For this review, take the finished solid that the model builds, in its own axes (mm). Face numbers are marked on the shaded views. A direction names the side the tool comes from. Coordinates: 2 decimals unless noted, no trailing zeros. Write each loop counter-clockwise with the first axis right and the second up, starting at its lowest first coordinate (ties: lowest second). Pieces come first, ordered by that corner, then holes.
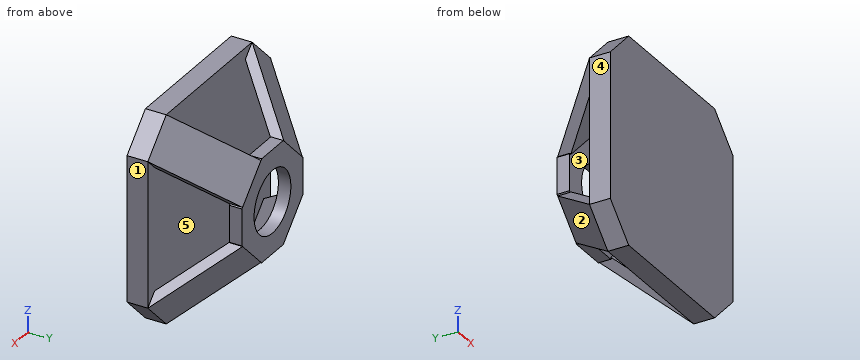
```python
from build123d import *
from build123d.topology import SkipClean

# Parameters (mm, degrees)
SKETCH1_W               = 20
SKETCH1_H               = 20
BOSS_EXTRUDE1_DEPTH     = 2
CHAMFER1_SIZE           = 3
EXTRUDE_THIN1_DEPTH     = 14.142136
CUT_EXTRUDE1_DEPTH      = 9.899495
CIRPATTERN5_START       = -2.121320344
CIRPATTERN5_DEPTH       = 4.242640688
CIRPATTERN5_START_2     = 12.02081528
CIRPATTERN5_2_DEPTH     = 4.242640687
CIRPATTERN5_START_3     = 2.121320344
CIRPATTERN5_3_OUTLINE_W = 4.242640688
CIRPATTERN5_3_OUTLINE_H = 2
CIRPATTERN5_3_DEPTH     = 9.899494936
SKETCH7_W               = 24.04163056
SKETCH7_H               = 24.04163056
CUT_EXTRUDE2_DEPTH      = 4
BOSS_EXTRUDE2_DEPTH     = 1.2
CHAMFER5_SIZE           = 2.5
CUT_EXTRUDE3_REACH      = 31.418
SKETCH10_R              = 3


with BuildPart() as part:
    # Sketch1 → Boss-Extrude1 (new body)
    with BuildSketch(Plane(origin=(0, 0, 0), x_dir=(1, 0, 0), z_dir=(0, 1, 0))):
        with Locations((10, 10)):
            Rectangle(SKETCH1_W, SKETCH1_H)
    extrude(amount=BOSS_EXTRUDE1_DEPTH)

    # Chamfer1
    chamfer1_edges = [part.edges().sort_by_distance(p)[0] for p in [
        (0, 1, -20),
        (20, 1, -20),
        (20, 1, 0),
        (0, 1, 0),
    ]]
    chamfer(chamfer1_edges, length=CHAMFER1_SIZE)



with BuildPart() as body_2:
    # Sketch3 → Extrude-Thin1 (new body)
    with BuildSketch(Plane(origin=(-8.5, 0, -8.5), x_dir=(-0.7071067811865488, 0, 0.7071067811865464), z_dir=(-0.7071067811865464, 0, -0.7071067811865488))):
        Polygon((-2.121320344, 2), (-14.142135624, 12.086661668), (-14.784923233, 11.320617225), (-2.764107953, 1.233955557), align=None)
    extrude(amount=-EXTRUDE_THIN1_DEPTH)

    # Sketch5 → Cut-Extrude1 (cut)
    with BuildSketch(Plane(origin=(-8.5, 0, -8.5), x_dir=(-0.7071067811865488, 0, 0.7071067811865462), z_dir=(-0.7071067811865462, 0, -0.7071067811865488))):
        Polygon((-2.121320344, 2), (-14.142135624, 12.086661668), (-14.784923233, 11.320617225), (-2.764107953, 1.233955557), align=None)
    extrude(amount=-CUT_EXTRUDE1_DEPTH, mode=Mode.SUBTRACT)


with BuildPart() as part_1:
    # CirPattern5: read off the stored shape, not the designer's step
    with SkipClean():  # the faces are left unmerged after this step: merging them gives an invalid solid
        add(part.part)

        add(body_2.part)  # CirPattern5 merges body 2
        # CirPattern5 outline → CirPattern5 (add)
        with BuildSketch(Plane(origin=(0, 0, 0), x_dir=(0.707106781186549, 0, -0.707106781186546), z_dir=(0.707106781186546, 0, 0.707106781186549)).offset(CIRPATTERN5_START)):
            Polygon((14.142135624, 10.781254379), (24.607227077, 2), (26.162950904, 2), (16.263455967, 10.306662551), (14.142135624, 12.086661668), (14.784923233, 11.320617225), align=None)
        extrude(amount=CIRPATTERN5_DEPTH)

    # CirPattern5 2 outline → CirPattern5 2 (add)
    with SkipClean():  # the faces are left unmerged after this step: merging them gives an invalid solid
        with BuildSketch(Plane(origin=(0, 0, 0), x_dir=(0.7071067811865541, 0, 0.707106781186541), z_dir=(0.707106781186541, 0, -0.707106781186554)).offset(CIRPATTERN5_START_2)):
            Polygon((0, -10.781254379), (-10.465091453, -2), (-12.02081528, -2), (-2.121320344, -10.30666255), (0, -12.086661668), (2.121320344, -10.30666255), (12.02081528, -2), (10.465091453, -2), align=None)
        extrude(amount=CIRPATTERN5_2_DEPTH)

    # CirPattern5 3 outline → CirPattern5 3 (add)
    with SkipClean():  # the faces are left unmerged after this step: merging them gives an invalid solid
        with BuildSketch(Plane(origin=(0, 0, 0), x_dir=(0.7071067811865541, 0, 0.707106781186541), z_dir=(0.707106781186541, 0, -0.707106781186554)).offset(CIRPATTERN5_START_3)):
            with Locations((0, -1)):
                Rectangle(CIRPATTERN5_3_OUTLINE_W, CIRPATTERN5_3_OUTLINE_H)
        extrude(amount=CIRPATTERN5_3_DEPTH)

    # Sketch7 → Cut-Extrude2 (cut)
    with BuildSketch(Plane(origin=(0, 12.086661668, 0), x_dir=(-0.7071067811865464, 0, -0.7071067811865488), z_dir=(0, 1, 0))):
        with Locations((0, -14.142135624)):
            Rectangle(SKETCH7_W, SKETCH7_H)
    extrude(amount=-CUT_EXTRUDE2_DEPTH, mode=Mode.SUBTRACT)

    # Sketch9 → Boss-Extrude2 (add)
    with BuildSketch(Plane(origin=(0, 8.086661668, 0), x_dir=(1, 0, 0), z_dir=(0, 1, 0))):
        Polygon((10, 16.741576375), (3.258423625, 10), (10, 3.258423625), (16.741576375, 10), align=None)
    extrude(amount=-BOSS_EXTRUDE2_DEPTH)

    # Chamfer5
    chamfer5_edges = [part_1.edges().sort_by_distance(p)[0] for p in [
        (10, 7.486661668, -3.258423625),
        (10, 7.486661668, -16.741576375),
        (16.741576375, 7.486661668, -10),
        (3.258423625, 7.486661668, -10),
    ]]
    chamfer(chamfer5_edges, length=CHAMFER5_SIZE)

    # Sketch10 → Cut-Extrude3 (cut, up to next)
    with BuildSketch(Plane(origin=(0, 8.086661668, 0), x_dir=(1, 0, 0), z_dir=(0, 1, 0)), mode=Mode.PRIVATE) as cut_extrude3_sk1:
        with Locations(Location((10, 10, 0), (0, 0, 270))):
            Circle(SKETCH10_R)
    cut_extrude3_tool1 = extrude(cut_extrude3_sk1.sketch, amount=-CUT_EXTRUDE3_REACH, mode=Mode.PRIVATE) & part_1.part
    add(cut_extrude3_tool1.solids().sort_by_distance((10, 8.086662, -10))[0], mode=Mode.SUBTRACT)


solid = part_1.part
```
Q1. Add section B-B (x = 10). State the section outline as (y, z) points, then the cut area to 3 significant figures.
Ans:
outline: (0, -20) - (2, -20) - (2, 0) - (0, 0) - close; (6.89, -14.97) - (8.09, -14.97) - (8.09, -13) - (6.89, -13) - close; (6.89, -7) - (8.09, -7) - (8.09, -5.03) - (6.89, -5.03) - close
area: 44.7 mm2
Q2. Draft analysis for pull direction Y (two halves, no side actions). For the marked faces 1, 2 and 3, state which applies: +Y half, -Y half, draft (parallel to the pull), parting line (faces both ways), or undercut.
Ans:
face 1: draft
face 2: +Y half
face 3: undercut
Q3. Add section D-D (z = -3.75). State the section outline as (x, y) points, then the cut area to 3 significant figures.
Ans:
outline: (0, 0) - (20, 0) - (20, 2) - (19.25, 2) - (19.25, 2.89) - (13.25, 6.45) - (13.25, 5.14) - (18.55, 2) - (1.45, 2) - (6.75, 5.14) - (6.75, 6.45) - (0.75, 2.89) - (0.75, 2) - (0, 2) - close
area: 55.4 mm2
Q4. Tool access review of the marked faces 4 and 5: name each direction out of +Z, -Z, +X, -X, +Y, -Y from which nothing blocks a thin tool from reaching the whole face with its end or side.
Ans:
face 4: +Z, -Z, -X, +Y, -Y
face 5: none
Q5. For probe 1 along X at (y, z) = (7.65, -10); probe 2 along Y at (x, z) = (10, -14); probe 3 along Y at (x, z) = (2, -8.75), list the stretches that pass through material, from the lowest coordinate up.
Ans:
probe 1: x = 5.03 to 7, 13 to 14.97
probe 2: y = 0 to 2, 6.89 to 8.09
probe 3: y = 0 to 2
Q6. Add section A-A (z = -10). State the section outline as (x, y) points.
Ans:
outline: (0, 0) - (20, 0) - (20, 2) - (0, 2) - close; (5.03, 6.89) - (7, 6.89) - (7, 8.09) - (5.03, 8.09) - close; (13, 6.89) - (14.97, 6.89) - (14.97, 8.09) - (13, 8.09) - close
Q7. Add section C-C (y = 3.75). State the section outline as (x, z) points, then the cut area to 3 significant figures.
Ans:
outline: (1.47, -15.53) - (4.47, -18.53) - (5.57, -17.43) - (2.57, -14.43) - close; (1.47, -4.47) - (2.57, -5.57) - (5.57, -2.57) - (4.47, -1.47) - close; (14.43, -17.43) - (15.53, -18.53) - (18.53, -15.53) - (17.43, -14.43) - close; (14.43, -2.57) - (17.43, -5.57) - (18.53, -4.47) - (15.53, -1.47) - close
area: 26.4 mm2
Q8. Clearance check with flat-ended pins moving along their axes: pin 1 Ø1.3 at (x, y) = (10.5, 7.5) entering from +Z; pin 2 Ø0.6 at (x, y) = (10, 7.5) entering from -Z; pin 3 Ø3.5 at (x, z) = (10, -10) entering from +Y. State where each tip first meets the part, or that it passes through.
Ans:
pin 1: stops at z = -5.03
pin 2: stops at z = -14.97
pin 3: stops at y = 2
